Work out the finished part from the listing and answer in its coordinate system (mm). Face numbers are marked on the shaded views. Coordinates: 2 decimals unless noted, no trailing zeros. Order: outer loops, then holes, each group sorted by start corner. A loop starts at its lowest first (then second) coordinate and runs counter-clockwise, first axis right, second up. Notation, with made-up numbers: M 25,-20.75 L 48,-20.75 A21 cw 48,-7.75 Z; hole C 73,85.25 d10. An arc over 180 degrees is marked long. Use a Markdown table: item, result.
from build123d import *

# Parameters (mm, degrees)
SKETCH_4_R               = 8
SKETCH_4_R_2             = 1.2
EXTRUDE_1_DEPTH          = 2
SKETCH_5_R               = 1.2
CUT_EXTRUDE_1_DEPTH      = 12.489125293
PATTERN_CIRCULAR_1_COUNT = 3


with BuildPart() as part:
    # 草图4 → 凸台-拉伸1 (new body)
    with BuildSketch(Plane(origin=(0, 0, 0), x_dir=(1, 0, 0), z_dir=(0, 1, 0))):
        with Locations(Location((0, 0, 0), (0, 0, 270))):
            Circle(SKETCH_4_R)
        with Locations(Location((0, 0, 0), (0, 0, 270))):
            Circle(SKETCH_4_R_2, mode=Mode.SUBTRACT)
    extrude(amount=EXTRUDE_1_DEPTH)

    # 草图5 → 切除-拉伸1 (cut, through all)
    with BuildSketch(Plane.XZ):
        with Locations(Location((0, 5, 0), (0, 0, 270))):
            Circle(SKETCH_5_R)
    cut_extrude_1 = extrude(amount=-CUT_EXTRUDE_1_DEPTH, mode=Mode.SUBTRACT)

    # 阵列(圆周)1: 切除-拉伸1 ×3 about axis
    pattern_circular_1_axis = Axis((0, 0, 0), (0, 1, 0))
    for i in range(1, PATTERN_CIRCULAR_1_COUNT):
        add(cut_extrude_1.rotate(pattern_circular_1_axis, i * 360 / PATTERN_CIRCULAR_1_COUNT), mode=Mode.SUBTRACT)


solid = part.part
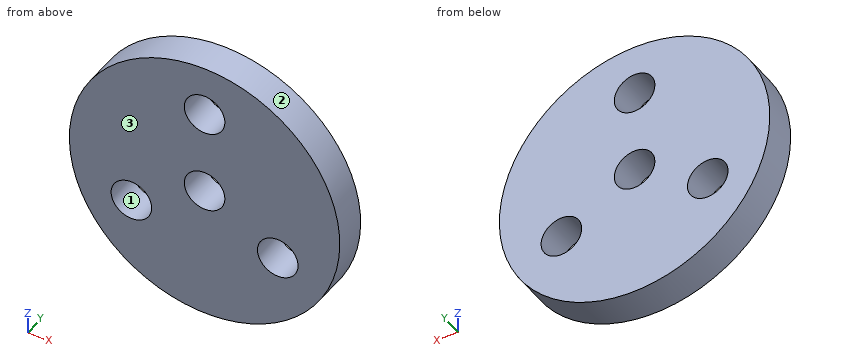
(1) A cutting plane is placed at D-D (x = -5.25). Determine the outline of the cut face in (y, z), then the cut area to 3 significant figures.
Conclusion:
| item | result |
|---|---|
| outline | M 0,-6.04 L 2,-6.04 L 2,-3.27 L 0,-3.27 Z; M 0,-1.73 L 2,-1.73 L 2,6.04 L 0,6.04 Z |
| area | 21.1 mm2 |
(2) Determine the mould class of the marked faces 1, 2 and 3 for opening direction Z: pulls with the +Z half, pulls with the -Z half, needs draft (parallel to the pull), parting line crosses it, or undercut.
Conclusion:
| item | result |
|---|---|
| face 1 | undercut |
| face 2 | parting line crosses it |
| face 3 | needs draft |
(3) A cutting plane is placed at B-B (x = 0). Determine the outline of the cut face in (y, z), then the cut area to 3 significant figures.
Conclusion:
| item | result |
|---|---|
| outline | M 0,-8 L 2,-8 L 2,-1.2 L 0,-1.2 Z; M 0,1.2 L 2,1.2 L 2,3.8 L 0,3.8 Z; M 0,6.2 L 2,6.2 L 2,8 L 0,8 Z |
| area | 22.4 mm2 |
(4) A cutting plane is placed at C-C (z = -2.75). Determine the outline of the cut face in (x, y), then the cut area to 3 significant figures.
Conclusion:
| item | result |
|---|---|
| outline | M -7.51,0 L -5.5,0 L -5.5,2 L -7.51,2 Z; M -3.16,0 L 3.16,0 L 3.16,2 L -3.16,2 Z; M 5.5,0 L 7.51,0 L 7.51,2 L 5.5,2 Z |
| area | 20.7 mm2 |
(5) Straight lines are drawn through the part: L1, parallel to X at y = 0.5, z = 0; L2, parallel to X at y = 0.9, z = -2.5; L3, parallel to X at y = 1.15, z = 5 (3 decimals). For each, find the intervals that lie inside material, in ascending order.
Conclusion:
| item | result |
|---|---|
| L1 | -8 to -1.2, 1.2 to 8 |
| L2 | -7.6 to -5.53, -3.13 to 3.13, 5.53 to 7.6 |
| L3 | -6.245 to -1.2, 1.2 to 6.245 |
(6) A cutting plane is placed at A-A (z = 0). Determine the outline of the cut face in (x, y).
Conclusion:
| item | result |
|---|---|
| outline | M -8,0 L -1.2,0 L -1.2,2 L -8,2 Z; M 1.2,0 L 8,0 L 8,2 L 1.2,2 Z |
(7) Given P1, Ø1, axis at x = -3.5, y = 1, coming from the -Z side, flat-ended and moving along its own axis, determine where the tip first touches the part or whether it passes through.
Conclusion:
| item | result |
|---|---|
| P1 | z = -7.42 |
